```python
from build123d import *

# Parameters (mm, degrees)
F0_W     = 101.6
F0_H     = 35.88385
F0_R     = 12.2174
F0_H_2   = 5.72135
F0_H_3   = 5.715
F1_DEPTH = 51.0794
F2_DEPTH = 63.5
F3_R     = 5.08


with BuildPart() as f1:
    # F0 (on Top) → F1 (new body)
    with BuildSketch(Plane.XY):
        with Locations((-23.954998, -38.374585)):
            Rectangle(F0_W, F0_H)
        with Locations((-23.954998, -38.37141)):
            Circle(F0_R, mode=Mode.SUBTRACT)
        with Locations((-23.954998, -17.571985)):
            Rectangle(F0_W, F0_H_2)
        with Locations((-23.954998, -59.17401)):
            Rectangle(F0_W, F0_H_3)
    extrude(amount=F1_DEPTH)

    # F0 (on Top) → F2 (join)
    with BuildSketch(Plane.XY):
        with BuildLine():
            ThreePointArc((26.522509, -8.99631), (-23.954998, 36.08869), (-74.432506, -8.99631))
            Line((-74.432506, -8.99631), (26.522509, -8.99631))
        make_face()
        with BuildLine():
            ThreePointArc((-74.432506, -8.99631), (-74.674311, -11.849264), (-74.754998, -14.71131))
            Line((-74.754998, -14.71131), (26.845002, -14.71131))
            ThreePointArc((26.845002, -14.71131), (26.764315, -11.849264), (26.522509, -8.99631))
            Line((26.522509, -8.99631), (-74.432506, -8.99631))
        make_face()
    extrude(amount=F2_DEPTH)

    # F3
    f3_edges = [f1.edges().sort_by_distance(p)[0] for p in [
        (-23.954998, -62.03151, 51.0794),
        (-23.954998, -14.71131, 51.0794),
        (-23.954998, -14.71131, 63.5),
        (26.845002, -62.03151, 25.5397),
        (-74.754998, -62.03151, 25.5397),
        (-23.954998, -62.03151, 0),
        (26.845002, -38.37141, 0),
    ]]
    fillet(f3_edges, radius=F3_R)


solid = f1.part
```
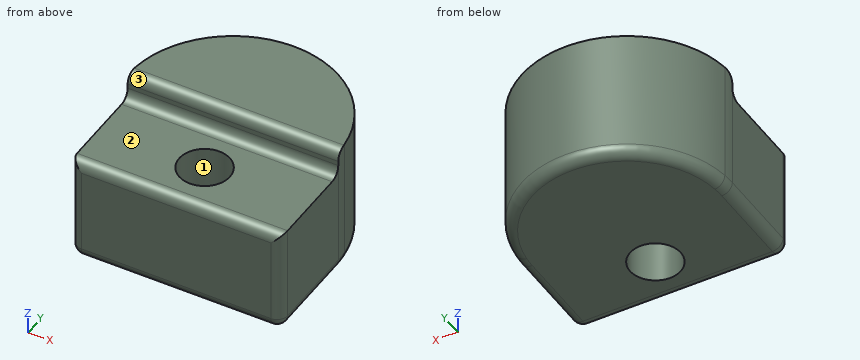
Read the model definition and answer for the solid it produces. Units are mm, in the model's axes. Face numbers are marked on the shaded views. Coordinates: 2 decimals unless noted, no trailing zeros. Loops run counter-clockwise (first coordinate to the right, second up) from the corner with the lowest first, then second, coordinate; pieces in that order, holes last. Notation, with made-up numbers: (71.25, -24) -> (128.25, -24) arc R20 ccw to (128.25, -14) -> close; hole circle Ø6 at (1.25, 69). An arc over 180 degrees is marked (long way). Return JSON: item names as keys, results as strings.
Item 1: Flat-ended cylindrical pins translate along their axes: P1, Ø10, axis at y = 16.5, z = 15.5, coming from the -X side; P2, Ø2, axis at x = -11.5, y = -23.5, coming from the +Z side; P3, Ø6, axis at x = -26, z = 39.5, coming from the +Y side; P4, Ø6, axis at x = -42, z = 7, coming from the +Y side. Find the tip coordinate at first contact, or state that the pin passes through.
Answers:
{"P1": "stops at x = -67.47", "P2": "stops at z = 51.08", "P3": "stops at y = 36.09", "P4": "stops at y = 33.81"}
Item 2: For a pull along Y with two mould halves and no side action, classify the marked faces 1, 2 and 3 as +Y half, -Y half, draft (parallel to the pull), parting line (faces both ways), or undercut.
Answers:
{"face 1": "undercut", "face 2": "draft", "face 3": "-Y half"}
Item 3: Find the intervals of material crossed by probe 1 along Y at (x, z) = (-18.5, 12); probe 2 along Y at (x, z) = (-30, 49.5); probe 3 along Y at (x, z) = (-46, 8), in increasing order.
Answers:
{"probe 1": "y = -62.03 to -49.3, -27.44 to 35.79", "probe 2": "y = -60.63 to -48.99, -27.75 to 35.73", "probe 3": "y = -62.03 to 31.06"}
Item 4: Find section D-D (y = -33). Determine the outline of the cut face in (x, z) (3 decimals).
Answers:
{"outline": "(-74.755, 5.08) arc R5.08 ccw to (-69.675, 0) -> (-34.928, 0) -> (-34.928, 51.079) -> (-74.755, 51.079) -> close; (-12.982, 0) -> (21.765, 0) arc R5.08 ccw to (26.845, 5.08) -> (26.845, 51.079) -> (-12.982, 51.079) -> close"}
Item 5: Find section B-B (z = 47.5). Determine the outline of the cut face in (x, y) (1 decimal).
Answers:
{"outline": "(-74.8, -57) arc R5.1 ccw to (-71.2, -61.8) -> (23.3, -61.8) arc R5.1 ccw to (26.8, -57) -> (26.8, -14.7) arc R50.8 ccw to (26.5, -9) arc R50.8 ccw to (-74.4, -9) arc R50.8 ccw to (-74.8, -14.7) -> close; hole circle Ø24.4 at (-24, -38.4)"}
Item 6: Find section C-C (z = 16). Determine the outline of the cut face in (x, y) (1 decimal), plus the area to 3 significant figures.
Answers:
{"outline": "(-74.8, -57) arc R5.1 ccw to (-69.7, -62) -> (21.8, -62) arc R5.1 ccw to (26.8, -57) -> (26.8, -14.7) arc R50.8 ccw to (26.5, -9) arc R50.8 ccw to (-74.4, -9) arc R50.8 ccw to (-74.8, -14.7) -> close; hole circle Ø24.4 at (-24, -38.4)", "area": "8,380 mm2"}
Item 7: Find section A-A (y = -44). Determine the outline of the cut face in (x, z) (3 decimals), plus the area to 3 significant figures.
Answers:
{"outline": "(-74.755, 5.08) arc R5.08 ccw to (-69.675, 0) -> (-34.799, 0) -> (-34.799, 51.079) -> (-74.755, 51.079) -> close; (-13.111, 0) -> (21.765, 0) arc R5.08 ccw to (26.845, 5.08) -> (26.845, 51.079) -> (-13.111, 51.079) -> close", "area": "4,070 mm2"}
